Check sheet for the modelled part. Datum: model origin and axes. Units: mm. Coordinates: 2 decimals unless noted, no trailing zeros. Order: outer loops, then holes, each group sorted by start corner. A loop starts at its lowest first (then second) coordinate and runs counter-clockwise, first axis right, second up.
from build123d import *

# Parameters (mm, degrees)
SKETCH_1_W           = 45
SKETCH_1_H           = 15
EXTRUDE_1_DEPTH      = 2.5
SKETCH_2_W           = 3
SKETCH_2_H           = 3
EXTRUDE_2_DEPTH      = 1
EXTRUDE_3_DEPTH      = 2
EXTRUDE_3_DEPTH_BACK = 2
CUT_EXTRUDE_1_DEPTH  = 41.234344782
FILLET_1_R           = 0.2
FILLET_2_R           = 0.1
EXTRUDE_4_DEPTH      = 2
CUT_EXTRUDE_2_DEPTH  = 10
FILLET_3_R           = 0.1


with BuildPart() as part:
    # 草图1 → 凸台-拉伸1 (new body)
    with BuildSketch(Plane.XY):
        Rectangle(SKETCH_1_W, SKETCH_1_H)
    extrude(amount=-EXTRUDE_1_DEPTH)

    # 草图2 → 凸台-拉伸2 (add)
    with BuildSketch(Plane.XY):
        with Locations((-15, 0)):
            Rectangle(SKETCH_2_W, SKETCH_2_H)
        with Locations((15, 0)):
            Rectangle(SKETCH_2_W, SKETCH_2_H)
    extrude(amount=EXTRUDE_2_DEPTH)

    # 草图3 → 凸台-拉伸3 (add, two sides: drawn at the far end of the back side and taken through both)
    with BuildSketch(Plane(origin=(0, 0, 0), x_dir=(1, 0, 0), z_dir=(0, 1, 0)).offset(-EXTRUDE_3_DEPTH_BACK)):
        with BuildLine():
            Line((-16.95, -2.5), (-13.05, -2.5))
            Line((-13.05, -2.5), (-13.05, -1.555590279))
            ThreePointArc((-13.05, -1.555590279), (-13.219957697, -1.088161527), (-13.5, -0.677124344))
            Line((-13.5, -0.677124344), (-16.5, -0.677124344))
            ThreePointArc((-16.5, -0.677124344), (-16.780042303, -1.088161527), (-16.95, -1.555590279))
            Line((-16.95, -1.555590279), (-16.95, -2.5))
        make_face()
        with BuildLine():
            Line((16.5, -0.677124344), (13.5, -0.677124344))
            ThreePointArc((13.5, -0.677124344), (13.219957697, -1.088161527), (13.05, -1.555590279))
            Line((13.05, -1.555590279), (13.05, -2.5))
            Line((13.05, -2.5), (16.95, -2.5))
            Line((16.95, -2.5), (16.95, -1.555590279))
            ThreePointArc((16.95, -1.555590279), (16.780042303, -1.088161527), (16.5, -0.677124344))
        make_face()
    extrude(amount=EXTRUDE_3_DEPTH + EXTRUDE_3_DEPTH_BACK)

    # 草图4 → 切除-拉伸1 (cut, through all)
    with BuildSketch(Plane.ZY.offset(16.95)):
        with BuildLine():
            Line((2.5, 1.95), (1.555590279, 1.95))
            ThreePointArc((1.555590279, 1.95), (1.088161527, 1.780042303), (0.677124344, 1.5))
            Line((0.677124344, 1.5), (0.677124344, 2))
            Line((0.677124344, 2), (2.5, 2))
            Line((2.5, 2), (2.5, 1.95))
        make_face()
        with BuildLine():
            Line((0.677124344, -2), (2.5, -2))
            Line((2.5, -2), (2.5, -1.95))
            Line((2.5, -1.95), (1.555590279, -1.95))
            ThreePointArc((1.555590279, -1.95), (1.088161527, -1.780042303), (0.677124344, -1.5))
            Line((0.677124344, -1.5), (0.677124344, -2))
        make_face()
    extrude(amount=-CUT_EXTRUDE_1_DEPTH, mode=Mode.SUBTRACT)

    # 圆角1
    fillet_1_edges = [part.edges().sort_by_distance(p)[0] for p in [
        (22.5, 0, -2.5),
        (0, 7.5, -2.5),
        (-22.5, 0, -2.5),
        (0, 7.5, 0),
        (22.5, 0, 0),
        (0, -7.5, 0),
        (-22.5, 0, 0),
        (0, -7.5, -2.5),
        (-22.5, 7.5, -1.25),
        (22.5, 7.5, -1.25),
        (22.5, -7.5, -1.25),
        (-22.5, -7.5, -1.25),
    ]]
    fillet(fillet_1_edges, radius=FILLET_1_R)

    # 圆角2
    fillet_2_edges = [part.edges().sort_by_distance(p)[0] for p in [
        (13.05, 0, 2.5),
        (16.95, 0, 2.5),
        (-16.95, 0, 2.5),
        (-13.05, 0, 2.5),
        (-15, -1.95, 2.5),
        (15, -1.95, 2.5),
        (-15, 1.95, 2.5),
        (15, 1.95, 2.5),
    ]]
    fillet(fillet_2_edges, radius=FILLET_2_R)

    # 草图6 → 凸台-拉伸4 (add, symmetric)
    with BuildSketch(Plane(origin=(0, 0, 0), x_dir=(1, 0, 0), z_dir=(0, 1, 0))):
        with BuildLine():
            Line((-6, 2.5), (-9, 2.5))
            Line((-9, 2.5), (-9, 3.177124344))
            ThreePointArc((-9, 3.177124344), (-9.280042303, 3.588161527), (-9.45, 4.055590279))
            Line((-9.45, 4.055590279), (-9.45, 5))
            Line((-9.45, 5), (-5.55, 5))
            Line((-5.55, 5), (-5.55, 4.055590279))
            ThreePointArc((-5.55, 4.055590279), (-5.719957697, 3.588161527), (-6, 3.177124344))
            Line((-6, 3.177124344), (-6, 2.5))
        make_face()
    extrude_4 = extrude(amount=EXTRUDE_4_DEPTH, both=True)

    # 草图7 → 切除-拉伸2 (cut)
    with BuildSketch(Plane(origin=(0, 0, 0), x_dir=(0, 0, -1), z_dir=(1, 0, 0))):
        with BuildLine():
            Line((2.5, 1.5), (3.177124344, 1.5))
            ThreePointArc((3.177124344, 1.5), (3.588161527, 1.780042303), (4.055590279, 1.95))
            Line((4.055590279, 1.95), (5, 1.95))
            Line((5, 1.95), (5, 2))
            Line((5, 2), (2.5, 2))
            Line((2.5, 2), (2.5, 1.5))
        make_face()
        with BuildLine():
            Line((5, -1.95), (4.055590279, -1.95))
            ThreePointArc((4.055590279, -1.95), (3.588161527, -1.780042303), (3.177124344, -1.5))
            Line((3.177124344, -1.5), (2.5, -1.5))
            Line((2.5, -1.5), (2.5, -2))
            Line((2.5, -2), (5, -2))
            Line((5, -2), (5, -1.95))
        make_face()
    cut_extrude_2 = extrude(amount=-CUT_EXTRUDE_2_DEPTH, mode=Mode.SUBTRACT)

    # 镜向1: 凸台-拉伸4, 切除-拉伸2 across plane
    add(extrude_4.mirror(Plane(origin=(0, 0, 0), x_dir=(0, 0, 1), z_dir=(1, 0, 0))))
    add(cut_extrude_2.mirror(Plane(origin=(0, 0, 0), x_dir=(0, 0, 1), z_dir=(1, 0, 0))), mode=Mode.SUBTRACT)

    # 圆角3
    fillet_3_edges = [part.edges().sort_by_distance(p)[0] for p in [
        (-5.55, 0, -5),
        (-9.45, 0, -5),
        (-7.5, -1.95, -5),
        (-7.5, 1.95, -5),
        (9.45, 0, -5),
        (5.55, 0, -5),
        (7.5, -1.95, -5),
        (7.5, 1.95, -5),
    ]]
    fillet(fillet_3_edges, radius=FILLET_3_R)


solid = part.part
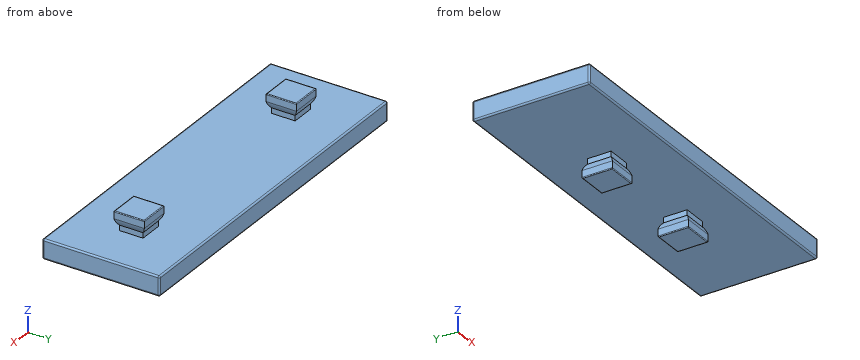
(1) Cross-section at B-B (y = 5). Enter the section's corners in (x, z), and give its area (3 significant figures).
Filled in:
outline: (-22.5, -2.3) arc R0.2 ccw to (-22.3, -2.5) - (22.3, -2.5) arc R0.2 ccw to (22.5, -2.3) - (22.5, -0.2) arc R0.2 ccw to (22.3, 0) - (-22.3, 0) arc R0.2 ccw to (-22.5, -0.2) - close
area: 112 mm2
(2) Thickness scan on probe 1 along Z at (x, y) = (12.5, -5); probe 2 along Y at (x, z) = (-7, -4.5); probe 3 along X at (y, z) = (0, 0.75). Record the ranges inside material, lowest first.
Filled in:
probe 1: z = -2.5 to 0
probe 2: y = -1.95 to 1.95
probe 3: x = -16.56 to -13.44, 13.44 to 16.56
(3) Go/stop test with flat-tipped pins: P1, Ø0.7, axis at x = -8, z = -4.5, coming from the +Y side; P2, Ø0.9, axis at x = -15.5, z = 2, coming from the +Y side; P3, Ø4.5, axis at x = -4.5, y = 3, coming from the +Z side; P4, Ø1.5, axis at y = -4, z = 1.5, coming from the +X side. Record where each tip stops, or that it passes through.
Filled in:
P1: stops at y = 1.95
P2: stops at y = 1.95
P3: stops at z = 0
P4: passes through
(4) Cross-section at A-A (x = 7.5). Enter the section's corners in (y, z), and give its area (3 significant figures).
Filled in:
outline: (-7.5, -2.3) arc R0.2 ccw to (-7.3, -2.5) - (-1.5, -2.5) - (-1.5, -3.18) arc R2 ccw to (-1.95, -4.06) - (-1.95, -4.9) arc R0.1 ccw to (-1.85, -5) - (1.85, -5) arc R0.1 ccw to (1.95, -4.9) - (1.95, -4.06) arc R2 ccw to (1.5, -3.18) - (1.5, -2.5) - (7.3, -2.5) arc R0.2 ccw to (7.5, -2.3) - (7.5, -0.2) arc R0.2 ccw to (7.3, 0) - (-7.3, 0) arc R0.2 ccw to (-7.5, -0.2) - close
area: 46.3 mm2
